Geometry: final body of the model. Coordinates: model frame, mm. A direction names the side the tool comes from. Round coordinates to 2 decimals unless told otherwise and drop trailing zeros. Write each loop counter-clockwise with the first axis right and the second up, starting at its lowest first coordinate (ties: lowest second). Pieces come first, ordered by that corner, then holes. Notation, with made-up numbers: M 3.25,31.5 L 37.25,31.5 A25 cw 37.25,60.5 Z; hole C 61.5,81 d3. An arc over 180 degrees is marked long. Answer as CSV lines item,"result". Start each with the question number.
Q1. Section query C-C on z = 29. Output: boundary loops of the cut face in (x, y), and give its area (3 significant figures).
Q2. Mould query, pull axis X, two halves, no side actions, for faces 1 (the flat face through (-15.721, 33, 44)), 2 (the flat face through (60.479, 33, 44)), 3 (the flat face through (22, 36.078, 38)), 4 (the flat face through (22, 11, 0)). Classes: pulls with the +X half, pulls with the -X half, needs draft (parallel to the pull), parting line crosses it, or undercut.
Q3. Section query B-B on y = 0. Output: boundary loops of the cut face in (x, z).
Q4. First-contact query: pin 1 (5.5 mm diameter, centred on x = -22, y = 24.5, fed in from +Z); pin 2 (12.5 mm diameter, centred on x = 28, z = 25.5, fed in from -Y); pin 3 (13.5 mm diameter, centred on x = 29.5, y = 7, fed in from +Z); pin 4 (2 mm diameter, centred on x = 50, y = -3, fed in from -Z). Flat tips, straight axial feed; report the tip coordinate or a pass-through.
Q5. Section query D-D on y = 33.5. Output: boundary loops of the cut face in (x, z).
Q6. Section query A-A on x = 17. Output: boundary loops of the cut face in (y, z), and give its area (3 significant figures).
Q7. Reachability of faces 5 (the flat face through (-27, 17, 38.1)), 6 (the flat face through (-9.371, 30, 38)), 7 (the flat face through (72, 17, 38.1)) from +Z, -Z, +X, -X, +Y, -Y: full face, straight path, thin tool, end or side. Return the list, or none.
Q8. Ray query, probe 1 along X at (y, z) = (35, 36); probe 2 along Z at (x, y) = (56, 6); probe 3 along Y at (x, z) = (18.5, 32). Return the intervals inside material, ascending.
```python
from build123d import *

# Parameters (mm, degrees)
F0_W     = 114.3
F0_H     = 63.5
F1_DEPTH = 38.1
F2_W     = 63.5
F2_H     = 6.35
F3_DEPTH = 12.7
F4_W     = 63.5
F4_H     = 12.7
F5_DEPTH = 12.7
F6_W     = 114.3
F6_H     = 12.7
F7_DEPTH = 25.4


with BuildPart() as f1:
    # F0 (on Top) → F1 (new body)
    with BuildSketch(Plane.XY):
        with Locations((22.379107, 10.678026)):
            Rectangle(F0_W, F0_H)
    extrude(amount=F1_DEPTH)

    # F2 (on face) → F3 (join)
    with BuildSketch(Plane.XY.offset(38.1)):
        Polygon((54.129107, 42.428026), (54.129107, 36.078026), (54.129107, 23.378026), (60.479107, 23.378026), (60.479107, 42.428026), align=None)
        with Locations((22.379107, 39.253026)):
            Rectangle(F2_W, F2_H)
        Polygon((-15.720893, 42.428026), (-15.720893, 23.378026), (-9.370893, 23.378026), (-9.370893, 36.078026), (-9.370893, 42.428026), align=None)
    extrude(amount=F3_DEPTH)

    # F4 (on face) → F5 (cut)
    with BuildSketch(Plane.XY.offset(38.1)):
        with Locations((22.379107, 29.728026)):
            Rectangle(F4_W, F4_H)
        Polygon((-15.720893, 23.378026), (-22.070893, 23.378026), (-22.070893, -8.371974), (66.829107, -8.371974), (66.829107, 23.378026), (60.479107, 23.378026), (54.129107, 23.378026), (-9.370893, 23.378026), align=None)
    extrude(amount=-F5_DEPTH, mode=Mode.SUBTRACT)

    # F6 (on face) → F7 (cut)
    with BuildSketch(Plane.XY.offset(38.1)):
        with Locations((22.379107, -14.721974)):
            Rectangle(F6_W, F6_H)
    extrude(amount=-F7_DEPTH, mode=Mode.SUBTRACT)


solid = f1.part
```
Entries:
1,outline,"M -34.77,-8.37 L -22.07,-8.37 L -22.07,23.38 L -9.37,23.38 L -9.37,36.08 L 54.13,36.08 L 54.13,23.38 L 66.83,23.38 L 66.83,-8.37 L 79.53,-8.37 L 79.53,42.43 L -34.77,42.43 Z"
1,area,"2,180 mm^2"
2,face 1,"pulls with the -X half"
2,face 2,"pulls with the +X half"
2,face 3,"undercut"
2,face 4,"needs draft"
3,outline,"M -34.77,0 L 79.53,0 L 79.53,38.1 L 66.83,38.1 L 66.83,25.4 L -22.07,25.4 L -22.07,38.1 L -34.77,38.1 Z"
4,pin 1,"stops at z = 38.1"
4,pin 2,"stops at y = -8.37"
4,pin 3,"stops at z = 25.4"
4,pin 4,"stops at z = 0"
5,outline,"M -34.77,0 L 79.53,0 L 79.53,38.1 L 60.48,38.1 L 60.48,50.8 L 54.13,50.8 L 54.13,25.4 L -9.37,25.4 L -9.37,50.8 L -15.72,50.8 L -15.72,38.1 L -34.77,38.1 Z"
6,outline,"M -21.07,0 L 42.43,0 L 42.43,50.8 L 36.08,50.8 L 36.08,25.4 L -8.37,25.4 L -8.37,12.7 L -21.07,12.7 Z"
6,area,"1,610 mm^2"
7,face 5,"+Z, -X, +Y, -Y"
7,face 6,"+Z, -Y"
7,face 7,"+Z, +X, +Y, -Y"
8,probe 1,"x = -34.77 to -9.37, 54.13 to 79.53"
8,probe 2,"z = 0 to 25.4"
8,probe 3,"y = 36.08 to 42.43"
